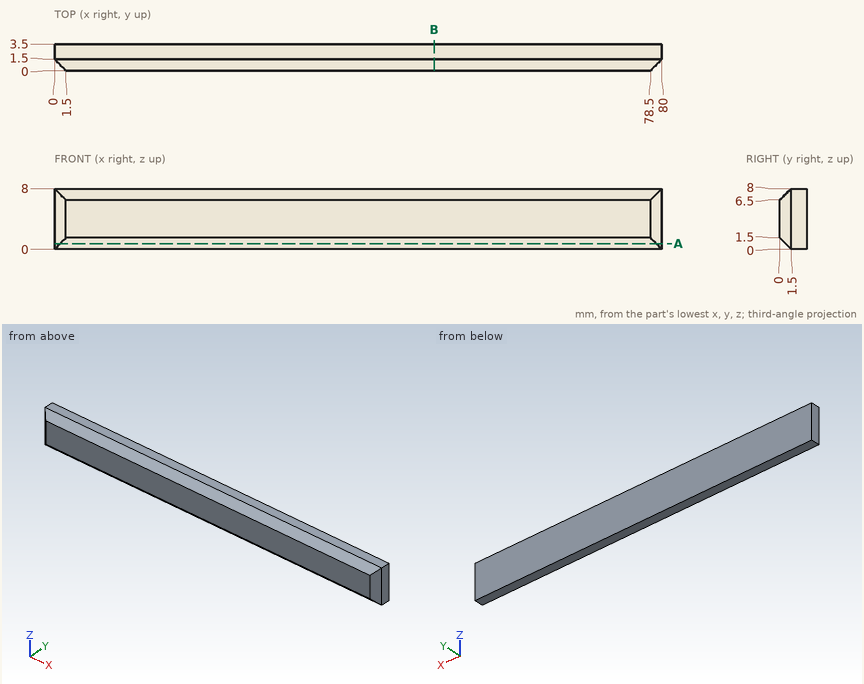
Source: three-view drawing plus pictorial views. Frame: mm from the lowest corner of the part. Round coordinates to 2 decimals unless told otherwise and drop trailing zeros. Loops run counter-clockwise (first coordinate to the right, second up) from the corner with the lowest first, then second, coordinate; pieces in that order, holes last.
Q1. Section A-A on z = 0.75. Return loops of the section in (x, y).
Q2. Section B-B on x = 50. Return loops of the section in (y, z).
Q3. Material intervals for L1, parallel to Z at x = 75, y = 0.8; L2, parallel to X at y = 1.3, z = 5; L3, parallel to Y at x = 47.5, z = 7.5, sorted ascending.
Evaluation:
1. outline: (0, 1.5) - (0.75, 0.75) - (79.25, 0.75) - (80, 1.5) - (80, 3.5) - (0, 3.5) - close
2. outline: (0, 1.5) - (1.5, 0) - (3.5, 0) - (3.5, 8) - (1.5, 8) - (0, 6.5) - close
3. L1: z = 0.7 to 7.3
3. L2: x = 0.2 to 79.8
3. L3: y = 1 to 3.5
